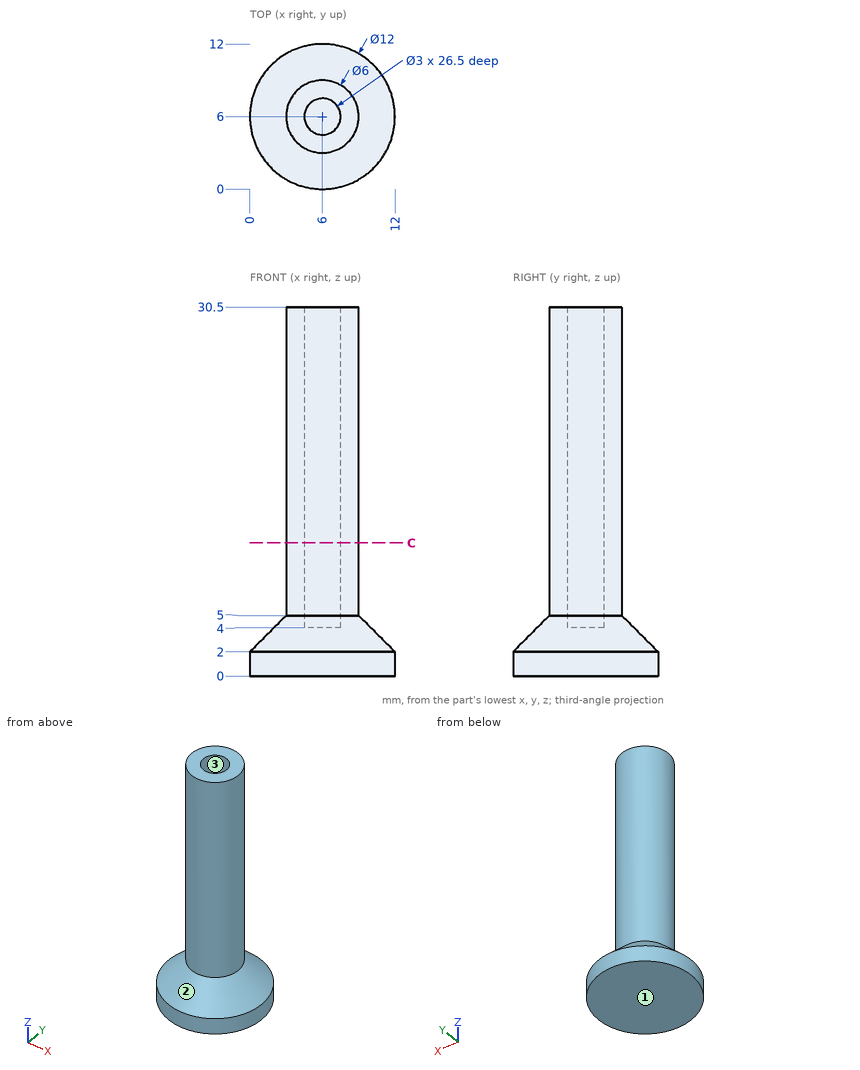
Design review of the part shown in the three views and the two pictorial views. Dimensions are in mm from the part's minimum x, y and z. Round coordinates to 2 decimals unless told otherwise and drop trailing zeros. Order: outer loops, then holes, each group sorted by start corner. A loop starts at its lowest first (then second) coordinate and runs counter-clockwise, first axis right, second up. Notation, with made-up numbers: (28, -14.75) -> (43, -14.75) arc R20 ccw to (43, -4.75) -> close; hole circle Ø4 at (-8.75, 19). An arc over 180 degrees is marked (long way). Write item = value, one per line. Start each with the question number.
1) To check wall thickness, follow line 1 (Y direction, x = 6, z = 20.75); line 2 (X direction, y = 7.25, z = 26.5); line 3 (X direction, y = 5, z = 4.5). State the ranges of each line that lie inside material, in increasing order. Write a range as from..to.
2) Take a section at C-C on z = 11. State the section outline as (x, y) points, plus the area to 3 significant figures.
3) Insertion check: pin 1 (3 mm diameter, centred on y = 9, z = 5.5, fed in from -X); pin 2 (6 mm diameter, centred on y = 3, z = 18, fed in from -X); pin 3 (4 mm diameter, centred on y = 8.5, z = 25.5, fed in from +X). Each pin has a flat end and moves straight along its axis. Give the tip position at first contact, or say it passes through.
4) The part is to be moulded in two halves that separate along Y. For the marked faces 1, 2 and 3, say which applies: +Y half, -Y half, draft (parallel to the pull), parting line (faces both ways), or undercut.
Verdict:
q1.line_1 = 3..4.5, 7.5..9
q1.line_2 = 3.27..5.17, 6.83..8.73
q1.line_3 = 2.65..4.88, 7.12..9.35
q2.outline = circle Ø6 at (6, 6); hole circle Ø3 at (6, 6)
q2.area = 21.2 mm2
q3.pin_1 = 2.94
q3.pin_2 = 3
q3.pin_3 = 8.96
q4.face_1 = draft
q4.face_2 = parting line
q4.face_3 = undercut
